Here's how the part is built. I have some questions about the finished solid (model axes, mm). A direction names the side the tool comes from. Round coordinates to 2 decimals unless told otherwise and drop trailing zeros. Loops run counter-clockwise (first coordinate to the right, second up) from the corner with the lowest first, then second, coordinate; pieces in that order, holes last. Notation, with made-up numbers: M 5.25,-7.75 L 23.25,-7.75 A27 ccw 23.25,30.25 Z; hole C -36.75,62.25 d1. An arc over 180 degrees is marked long. Use a Markdown table: item, result.
Autodesk Inventor part; units mm, degrees
ref_plane "YZ Plane" through (0, 0, 0) normal (1, 0, 0) x (0, 1, 0)
ref_plane "XZ Plane" through (0, 0, 0) normal (0, 1, 0) x (-1, 0, 0)
ref_plane "XY Plane" through (0, 0, 0) normal (0, 0, 1) x (1, 0, 0)
sketch "草图1" plane through (0, 0, 0) normal (0, 0, 1) x (1, 0, 0)
  line L0 (0, 0) -> (1.4, 0)
  line L1 (1.4, -3) -> (0, -3)
  line L2 (0, 0) -> (-3, 0)
  line L3 (-3, -7) -> (0, -7)
  line L4 (0, -7) -> (0, -3)
  line L5 (-5, -4.6) -> (-5, -1)
  line L6 (-5, -1) -> (-3, -1)
  line L7 (-3, -6.9664) -> (-3, -7)
  arc A0 (-5, -4.6) -> (-2.6, -7) centre (-2.6, -4.6) ccw
  line L8 (1.4, -3) -> (3.1321, -4)
  line L9 (-3, 0) -> (-3, -1)
  line L10 (-3, -6.9664) -> (-3, -7)
  line L11 (1.4, 0) -> (26.7321, 0)
  line L12 (26.7321, 0) -> (26.7321, -4)
  line L13 (26.7321, -4) -> (3.1321, -4)
  dimension "d0" = 1.4
  dimension "d1" = 3
  dimension "d2" = 3
  dimension "d4" = 2
  dimension "d6" = 4.8
  dimension "d7" = 30
  dimension "d9" = 23.6
  dimension "d10" = 4
revolve "旋转1" add sketch "草图1" angle 360 about axis through (1.4, 0, 0) along (1, 0, 0) contours L0 L11 L12 L13 L8 L1 L4 L3 A0 L5 L6 L9 L2
properties part number "13-螺钉" material "不锈钢"
1. I need wall thicknesses on probe 1 along Y at (x, z) = (-3.4, 0); probe 2 along Y at (x, z) = (-4.05, 0); probe 3 along Z at (x, y) = (-3.75, 0). Which ranges of each line are inside material? Lowest first, please. Write a range as from..to.
Answer sheet:
| item | result |
|---|---|
| probe 1 | -6.86..-1, 1..6.86 |
| probe 2 | -6.51..-1, 1..6.51 |
| probe 3 | -6.71..-1, 1..6.71 |
2. Imagine slicing it at C-C, the plane x = 25. Write out the boundary of the cut face in (y, z).
Answer sheet:
| item | result |
|---|---|
| outline | C 0,0 d8 |
3. For pin 1 Ø6 at (x, y) = (11.5, 1) entering from +Z; pin 2 Ø1.2 at (y, z) = (0, 0) entering from -X; pin 3 Ø4 at (x, z) = (2.5, 5) entering from -Y, each with a flat end and sliding along its axis, tell me the tip position at first contact or that it passes through.
Answer sheet:
| item | result |
|---|---|
| pin 1 | z = 4 |
| pin 2 | x = -3 |
| pin 3 | y = -2.52 |
4. Imagine slicing it at A-A, the plane z = 0. Write out the boundary of the cut face in (x, y), then the cut area to 3 significant figures.
Answer sheet:
| item | result |
|---|---|
| outline | M -5,-4.6 A2.4 ccw -2.6,-7 L 0,-7 L 0,-3 L 1.4,-3 L 3.13,-4 L 26.73,-4 L 26.73,4 L 3.13,4 L 1.4,3 L 0,3 L 0,7 L -2.6,7 A2.4 ccw -5,4.6 L -5,1 L -3,1 L -3,-1 L -5,-1 Z |
| area | 273 mm2 |
5. We'd pull the mould along Z, two halves only. Please class faces 5 (the face through (-5, -1, 1)), 6 (the face through (-4, 0, 1)), 7 (the face through (1, 3, 0)): +Z half, -Z half, draft (parallel to the pull), parting line (faces both ways), or undercut.
Answer sheet:
| item | result |
|---|---|
| face 5 | draft |
| face 6 | undercut |
| face 7 | parting line |
6. Which directions (+Z, -Z, +X, -X, +Y, -Y) give clear straight access to the entire face, cutting with the end or side of a thin tool? Please do faces 1 (the face through (14.767, 0.867, -3.905)), 2 (the face through (-3, 0, 0)), 3 (the face through (0, -1, 3)), 4 (the face through (-1.282, -6.466, 2.681)).
Answer sheet:
| item | result |
|---|---|
| face 1 | +X |
| face 2 | -X |
| face 3 | none |
| face 4 | +X, -X |
